```python
from build123d import *

# Parameters (mm, degrees)
SKETCH1_R                = 40
BOSS_EXTRUDE1_DEPTH      = 27
SKETCH2_R                = 3
CUT_EXTRUDE1_DEPTH       = 1
CUT_EXTRUDE1_DEPTH_BACK  = 45
SKETCH3_R                = 18.5
SKETCH3_R_2              = 8.5
CUT_EXTRUDE2_DEPTH       = 23
SKETCH4_R                = 23.5
SKETCH4_R_2              = 18.5
CUT_EXTRUDE5_DEPTH       = 19
SKETCH6_R                = 40
SKETCH6_R_2              = 22.5
CUT_EXTRUDE6_DEPTH       = 4
SKETCH7_R                = 40
SKETCH7_R_2              = 27.5
CUT_EXTRUDE7_DEPTH       = 12
SKETCH8_R                = 35
SKETCH8_R_2              = 8.5
CUT_EXTRUDE8_DEPTH       = 8.5
SKETCH9_R                = 24.75
SKETCH9_R_2              = 8.5
CUT_EXTRUDE13_DEPTH      = 0.95
SKETCH10_R               = 3
CUT_EXTRUDE14_DEPTH      = 13
CUT_EXTRUDE14_DEPTH_BACK = 16
SKETCH11_R               = 2
CUT_EXTRUDE22_DEPTH      = 11
SKETCH12_R               = 4
CUT_EXTRUDE23_DEPTH      = 1
CIRPATTERN1_COUNT        = 6
CUT_EXTRUDE24_REACH      = 42
SKETCH13_R               = 1.5
SKETCH14_R               = 40
SKETCH14_R_2             = 27
CUT_EXTRUDE25_DEPTH      = 7
CUT_EXTRUDE26_REACH      = 42
SKETCH15_R               = 1.5
SKETCH16_R               = 8.5
BOSS_EXTRUDE2_DEPTH      = 4.1
SKETCH17_R               = 8.5
SKETCH17_R_2             = 7.5
CUT_EXTRUDE27_DEPTH      = 8
SKETCH18_R               = 3
CUT_EXTRUDE28_DEPTH      = 7


with BuildPart() as part:
    # Sketch1 → Boss-Extrude1 (new body)
    with BuildSketch(Plane(origin=(0, 0, 0), x_dir=(0, 0, -1), z_dir=(1, 0, 0))):
        Circle(SKETCH1_R)
    extrude(amount=BOSS_EXTRUDE1_DEPTH)

    # Sketch2 → Cut-Extrude1 (cut, two sides)
    with BuildSketch(Plane.ZY) as cut_extrude1_sk:
        Circle(SKETCH2_R)
    extrude(amount=CUT_EXTRUDE1_DEPTH, mode=Mode.SUBTRACT)
    extrude(cut_extrude1_sk.sketch, amount=-CUT_EXTRUDE1_DEPTH_BACK, mode=Mode.SUBTRACT)

    # Sketch3 → Cut-Extrude2 (cut)
    with BuildSketch(Plane(origin=(27, 0, 0), x_dir=(0, 0, -1), z_dir=(1, 0, 0))):
        Circle(SKETCH3_R)
        Circle(SKETCH3_R_2, mode=Mode.SUBTRACT)
    extrude(amount=-CUT_EXTRUDE2_DEPTH, mode=Mode.SUBTRACT)

    # Sketch4 → Cut-Extrude5 (cut)
    with BuildSketch(Plane(origin=(27, 0, 0), x_dir=(0, 0, -1), z_dir=(1, 0, 0))):
        Circle(SKETCH4_R)
        Circle(SKETCH4_R_2, mode=Mode.SUBTRACT)
    extrude(amount=-CUT_EXTRUDE5_DEPTH, mode=Mode.SUBTRACT)

    # Sketch6 → Cut-Extrude6 (cut)
    with BuildSketch(Plane.ZY):
        Circle(SKETCH6_R)
        Circle(SKETCH6_R_2, mode=Mode.SUBTRACT)
    extrude(amount=-CUT_EXTRUDE6_DEPTH, mode=Mode.SUBTRACT)

    # Sketch7 → Cut-Extrude7 (cut)
    with BuildSketch(Plane(origin=(27, 0, 0), x_dir=(0, 0, -1), z_dir=(1, 0, 0))):
        Circle(SKETCH7_R)
        Circle(SKETCH7_R_2, mode=Mode.SUBTRACT)
    extrude(amount=-CUT_EXTRUDE7_DEPTH, mode=Mode.SUBTRACT)

    # Sketch8 → Cut-Extrude8 (cut)
    with BuildSketch(Plane(origin=(27, 0, 0), x_dir=(0, 0, -1), z_dir=(1, 0, 0))):
        Circle(SKETCH8_R)
        Circle(SKETCH8_R_2, mode=Mode.SUBTRACT)
    extrude(amount=-CUT_EXTRUDE8_DEPTH, mode=Mode.SUBTRACT)

    # Sketch9 → Cut-Extrude13 (cut, symmetric)
    with BuildSketch(Plane(origin=(15.95, 0, 0), x_dir=(0, 0, -1), z_dir=(1, 0, 0))):
        Circle(SKETCH9_R)
        Circle(SKETCH9_R_2, mode=Mode.SUBTRACT)
    extrude(amount=CUT_EXTRUDE13_DEPTH, both=True, mode=Mode.SUBTRACT)

    # Sketch10 → Cut-Extrude14 (cut, two sides)
    with BuildSketch(Plane(origin=(15, 0, 0), x_dir=(0, 0, -1), z_dir=(1, 0, 0))) as cut_extrude14_sk:
        with Locations((20.032335111, 20.032335111)):
            Circle(SKETCH10_R)
    extrude(amount=CUT_EXTRUDE14_DEPTH, mode=Mode.SUBTRACT)
    extrude(cut_extrude14_sk.sketch, amount=-CUT_EXTRUDE14_DEPTH_BACK, mode=Mode.SUBTRACT)

    # Sketch11 → Cut-Extrude22 (cut)
    with BuildSketch(Plane(origin=(15, 0, 0), x_dir=(0, 0, -1), z_dir=(1, 0, 0))):
        with Locations((33, 0)):
            Circle(SKETCH11_R)
    cut_extrude22 = extrude(amount=-CUT_EXTRUDE22_DEPTH, mode=Mode.SUBTRACT)

    # Sketch12 → Cut-Extrude23 (cut)
    with BuildSketch(Plane(origin=(15, 0, 0), x_dir=(0, 0, -1), z_dir=(1, 0, 0))):
        with Locations((33, 0)):
            Circle(SKETCH12_R)
    cut_extrude23 = extrude(amount=-CUT_EXTRUDE23_DEPTH, mode=Mode.SUBTRACT)

    # CirPattern1: Cut-Extrude22, Cut-Extrude23 ×6 about axis
    cirpattern1_axis = Axis((0, 0, 0), (1, 0, 0))
    for i in range(1, CIRPATTERN1_COUNT):
        add(cut_extrude22.rotate(cirpattern1_axis, i * 360 / CIRPATTERN1_COUNT), mode=Mode.SUBTRACT)
        add(cut_extrude23.rotate(cirpattern1_axis, i * 360 / CIRPATTERN1_COUNT), mode=Mode.SUBTRACT)

    # Sketch13 → Cut-Extrude24 (cut, up to next)
    with BuildSketch(Plane(origin=(0, 0, 0), x_dir=(1, 0, 0), z_dir=(0, 1, 0)), mode=Mode.PRIVATE) as cut_extrude24_sk1:
        with Locations((21, 0)):
            Circle(SKETCH13_R)
    cut_extrude24_tool1 = extrude(cut_extrude24_sk1.sketch, amount=CUT_EXTRUDE24_REACH, mode=Mode.PRIVATE) & part.part
    add(cut_extrude24_tool1.solids().sort_by_distance((21, 0, 0))[0], mode=Mode.SUBTRACT)

    # Sketch14 → Cut-Extrude25 (cut)
    with BuildSketch(Plane.ZY.offset(-4)):
        Circle(SKETCH14_R)
        Circle(SKETCH14_R_2, mode=Mode.SUBTRACT)
    extrude(amount=-CUT_EXTRUDE25_DEPTH, mode=Mode.SUBTRACT)

    # Sketch15 → Cut-Extrude26 (cut, up to next)
    with BuildSketch(Plane.XY, mode=Mode.PRIVATE) as cut_extrude26_sk1:
        with Locations((21, 0)):
            Circle(SKETCH15_R)
    cut_extrude26_tool1 = extrude(cut_extrude26_sk1.sketch, amount=-CUT_EXTRUDE26_REACH, mode=Mode.PRIVATE) & part.part
    add(cut_extrude26_tool1.solids().sort_by_distance((21, 0, 0))[0], mode=Mode.SUBTRACT)

    # Sketch16 → Boss-Extrude2 (add)
    with BuildSketch(Plane(origin=(27, 0, 0), x_dir=(0, 0, -1), z_dir=(1, 0, 0))):
        Circle(SKETCH16_R)
    extrude(amount=BOSS_EXTRUDE2_DEPTH)

    # Sketch17 → Cut-Extrude27 (cut)
    with BuildSketch(Plane(origin=(31.1, 0, 0), x_dir=(0, 0, -1), z_dir=(1, 0, 0))):
        Circle(SKETCH17_R)
        Circle(SKETCH17_R_2, mode=Mode.SUBTRACT)
    extrude(amount=-CUT_EXTRUDE27_DEPTH, mode=Mode.SUBTRACT)

    # Sketch18 → Cut-Extrude28 (cut)
    with BuildSketch(Plane(origin=(31.1, 0, 0), x_dir=(0, 0, -1), z_dir=(1, 0, 0))):
        Circle(SKETCH18_R)
    extrude(amount=-CUT_EXTRUDE28_DEPTH, mode=Mode.SUBTRACT)


solid = part.part
```
Build history of the part. All positions in model axes, mm. A direction names the side the tool comes from. Coordinates: 2 decimals unless noted, no trailing zeros. Order: outer loops, then holes, each group sorted by start corner. A loop starts at its lowest first (then second) coordinate and runs counter-clockwise, first axis right, second up.
Item 1: Saw through at B-B on x = 21. List the corners of the cut face in (y, z).
Filled in:
outline: (-1.5, -8.37) - (-1.5, -2.6) arc R3 cw (long way) to (2.6, 1.5) - (8.37, 1.5) arc R8.5 ccw (long way) to start; (1.5, -8.37) arc R8.5 ccw to (8.37, -1.5) - (2.6, -1.5) arc R3 cw to (1.5, -2.6) - close
Item 2: Drop flat-ended pins along their axis: pin 1 Ø6 at (y, z) = (-14, -8) entering from +X; pin 2 Ø6.5 at (y, z) = (-28.58, -16.5) entering from +X; pin 3 Ø4 at (y, z) = (-31.5, -12.5) entering from +X. Give the stop position or say it passes through.
Filled in:
pin 1: stops at x = 8
pin 2: stops at x = 14
pin 3: stops at x = 15
Item 3: Drill centre lines: L1, parallel to X at y = 4.8, z = 0; L2, parallel to Z at x = 12.5, y = 30; L3, parallel to Y at x = 12, z = 16. Where is each one in solid material? Low to high.
Filled in:
L1: x = 0 to 19.5, 22.5 to 31.1
L2: z = -26.46 to -17.91, -15.09 to 15.09, 17.91 to 26.46
L3: y = -36.66 to -30.52, -26.64 to -17.21, 17.21 to 26.64, 30.52 to 36.66
Item 4: Tool access for faces 1 (the flat face through (14, -28, -19)), 2 (the cylindrical face through (19.5, 0.07, -5.51)), 3 (the flat face through (4, -22, 6)): list every direction of +Z, -Z, +X, -X, +Y, -Y with a clear straight run to the whole face (end or side of a thin tool).
Filled in:
face 1: +X
face 2: -Z
face 3: -X
Item 5: Mould opens along Z. For faces 4 (the cylindrical face through (12.521, -26.626, -16.934)), 5 (the cylindrical face through (1.972, -19.961, 10.382)), 6 (the flat face through (0, -5, 0)) say: released by +Z, released by -Z, zero draft, split by the parting line, or undercut.
Filled in:
face 4: undercut
face 5: split by the parting line
face 6: zero draft
Item 6: Saw through at A-A on z = 33. List the corners of the cut face in (x, y), then the cut area to 3 significant figures.
Filled in:
outline: (11, -22.61) - (15, -22.61) - (15, -4) - (14, -4) - (14, -2) - (11, -2) - close; (11, 2) - (14, 2) - (14, 4) - (15, 4) - (15, 22.61) - (11, 22.61) - close
area: 161 mm2
